Input: part model. Units: mm. Frame: model coordinates. A direction names the side the tool comes from. Give positions to 0.01 mm unless a question says otherwise; leave off trailing zeros. Order: outer loops, then holes, each group sorted by start corner. A loop starts at its lowest first (then second) coordinate and runs counter-clockwise, first axis right, second up. Notation, with made-up numbers: M 40,-0.5 L 49,-0.5 A25 ccw 49,15.5 Z; hole C 77.25,87.25 d11. An arc over 180 degrees is marked long. Use a Markdown table: item, result.
from build123d import *

# Parameters (mm, degrees)
F1_DEPTH  = 150
F2_R      = 16.5902207369
F3_DEPTH  = 30
F3_FACE_R = 16.5902207369
F4_DEPTH  = 15
F4_TAPER  = -65


with BuildPart() as f1:
    # F0 (on Front) → F1 (new body)
    with BuildSketch(Plane.XZ):
        Polygon((-5.0131896813, -17.1994746155), (7.2152830783, -16.3979781659), (16.0676446966, -7.9236854892), (17.4017767894, 4.2581876898), (10.5934241232, 14.4476075243), (-1.171709423, 17.8768312309), (-12.3885871081, 12.9412869257), (-17.8087072015, 1.9503706416), (-14.8959352736, -9.9531457416), align=None)
    extrude(amount=F1_DEPTH)

    # F2 (on Front) → F3 (join)
    with BuildSketch(Plane.XZ):
        Circle(F2_R)
    extrude(amount=-F3_DEPTH)

    # F3_face (on face) → F4 (join)
    with BuildSketch(Plane(origin=(0, 30, 0), x_dir=(1, 0, 0), z_dir=(0, 1, 0))):
        Circle(F3_FACE_R)
    extrude(amount=F4_DEPTH, taper=F4_TAPER)


solid = f1.part
1) First-contact query: pin 1 Ø10 at (x, z) = (16, -23.5) entering from -Y; pin 2 Ø12 at (y, z) = (-17.5, -7) entering from -X; pin 3 Ø8 at (y, z) = (-37, 12.5) entering from +X. Flat tips, straight axial feed; report the tip coordinate or a pass-through.
Response values:
| item | result |
|---|---|
| pin 1 | stops at y = 33.19 |
| pin 2 | stops at x = -17.09 |
| pin 3 | stops at x = 14.57 |
2) Mould query, pull axis Y, two halves, no side actions, for faces 1 (the face through (-16.574, 14.79, 0.729)), 2 (the face through (4.79, -73.95, 16.14)), 3 (the face through (0, -150, 1)), 4 (the face through (-1, 45, -1)). Classes: released by +Y, released by -Y, zero draft, split by the parting line, or undercut.
Response values:
| item | result |
|---|---|
| face 1 | undercut |
| face 2 | zero draft |
| face 3 | released by -Y |
| face 4 | released by +Y |
3) Material intervals for line 1 (X direction, y = -91.5, z = -8); line 2 (Y direction, x = 34.5, z = -17); line 3 (Y direction, x = 43, z = 13), sorted ascending. Write a range as from..to.
Response values:
| item | result |
|---|---|
| line 1 | x = -15.37..15.99 |
| line 2 | y = 40.2..45 |
| line 3 | y = 43.21..45 |
4) Reachability of faces 5 (the face through (-6.702, -73.95, 15.444)), 6 (the face through (-10.02, -73.95, -13.53)), 7 (the face through (14.045, -73.95, 9.282)) from +Z, -Z, +X, -X, +Y, -Y: full face, straight path, thin tool, end or side. Return the list, or none.
Response values:
| item | result |
|---|---|
| face 5 | +Z, -X, -Y |
| face 6 | -Z, -X, -Y |
| face 7 | +Z, +X, -Y |
5) Cut plane A-A on y = -62.5. Return loops of the section in (x, z), and give its area (3 significant figures).
Response values:
| item | result |
|---|---|
| outline | M -17.81,1.95 L -14.9,-9.95 L -5.01,-17.2 L 7.22,-16.4 L 16.07,-7.92 L 17.4,4.26 L 10.59,14.45 L -1.17,17.88 L -12.39,12.94 Z |
| area | 928 mm² |
6) Cut plane B-B on y = 8. Return loops of the section in (x, z), and give its area (3 significant figures).
Response values:
| item | result |
|---|---|
| outline | C 0,0 d33.18 |
| area | 865 mm² |
